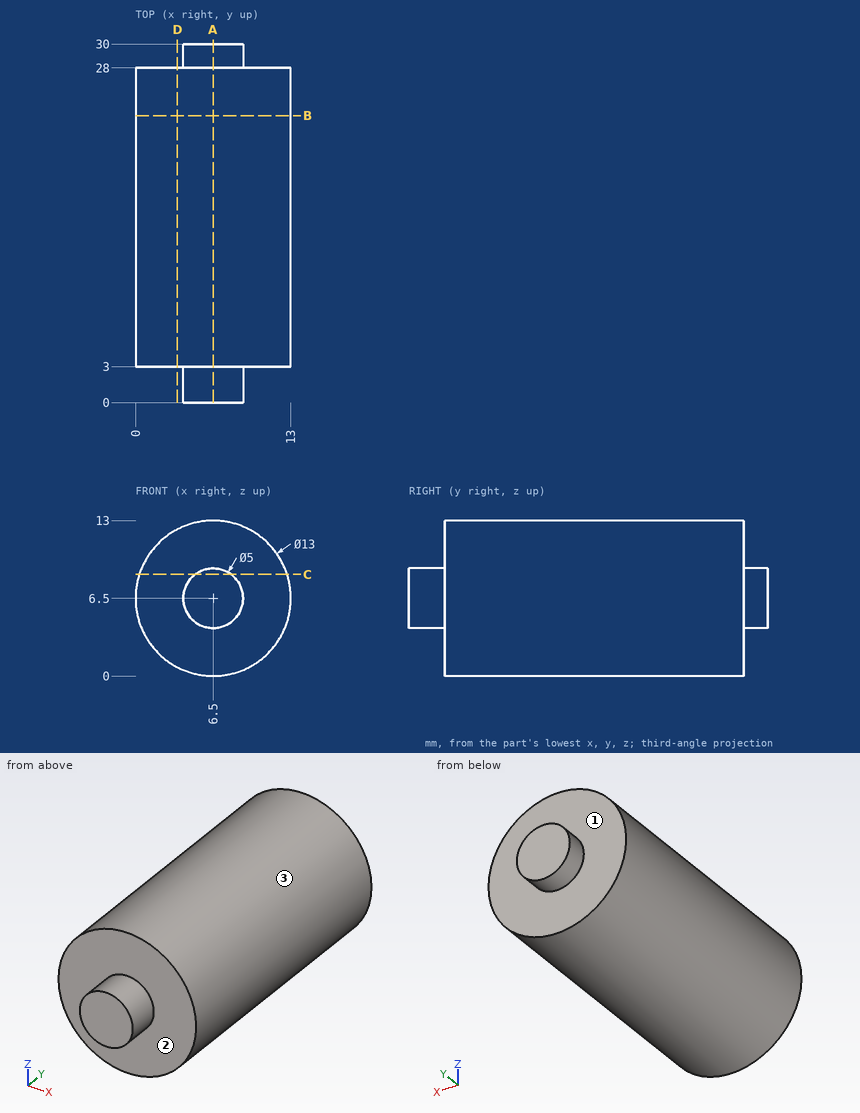
Study the drawing (mm; zero at the part's minimum x, y, z) and answer. A direction names the side the tool comes from. Give positions to 0.01 mm unless a question says otherwise; leave off trailing zeros. Write each loop counter-clockwise with the first axis right and the second up, starting at its lowest first coordinate (ties: lowest second). Pieces come first, ordered by that corner, then holes. Notation, with made-up numbers: (67.25, 89.25) -> (105.25, 89.25) arc R10 cw to (105.25, 97.25) -> close; hole circle Ø4 at (60.5, 88). An arc over 180 degrees is marked (long way). Write item = value, one per line.
Q1. Section C-C on z = 8.5 is taken. Determine the outline of the cut face in (x, y), and give its area (3 significant figures).
Computed values:
outline = (0.32, 3) -> (5, 3) -> (5, 0) -> (8, 0) -> (8, 3) -> (12.68, 3) -> (12.68, 28) -> (8, 28) -> (8, 30) -> (5, 30) -> (5, 28) -> (0.32, 28) -> close
area = 324 mm^2
Q2. Section A-A on x = 6.5 is taken. Determine the outline of the cut face in (y, z).
Computed values:
outline = (0, 4) -> (3, 4) -> (3, 0) -> (28, 0) -> (28, 4) -> (30, 4) -> (30, 9) -> (28, 9) -> (28, 13) -> (3, 13) -> (3, 9) -> (0, 9) -> close
Q3. Consider line 1 along Y through (x, z) = (3.75, 8.5); line 2 along Z through (x, y) = (6.25, 19.75); line 3 along Z through (x, y) = (6, 29.25). Determine where each line is inside the solid, lowest interval first.
Computed values:
line_1 = 3 to 28
line_2 = 0 to 13
line_3 = 4.05 to 8.95
Q4. A tool of negligible diameter and unlimited length cuts with its end or side. For the marked faces 1, 2 and 3, from which of +Z, -Z, +X, -X, +Y, -Y can it reach the whole face along a straight path? Write none if from no direction.
Computed values:
face_1 = +Y
face_2 = -Y
face_3 = +Y, -Y
Q5. Section B-B on y = 24 is taken. Determine the outline of the cut face in (x, z), and give its area (3 significant figures).
Computed values:
outline = circle Ø13 at (6.5, 6.5)
area = 133 mm^2
Q6. Section D-D on x = 3.5 is taken. Determine the outline of the cut face in (y, z), and give its area (3 significant figures).
Computed values:
outline = (3, 0.73) -> (28, 0.73) -> (28, 12.27) -> (3, 12.27) -> close
area = 288 mm^2
Q7. Flat-ended cylindrical pins translate along their axes: pin 1 Ø5 at (x, y) = (5, 19.5) entering from -Z; pin 2 Ø1.5 at (x, z) = (2, 9) entering from +Y; pin 3 Ø4 at (y, z) = (18, 10.5) entering from -X. Find the tip coordinate at first contact, or state that the pin passes through.
Computed values:
pin_1 = 0
pin_2 = 28
pin_3 = 0.32
